Part model, mm, in its own coordinate system. Give positions to 0.01 mm unless a question says otherwise; leave off trailing zeros. Order: outer loops, then holes, each group sorted by start corner. A loop starts at its lowest first (then second) coordinate and runs counter-clockwise, first axis right, second up.
1. Slice it at A-A on z = 26. List the corners of the cut face in (x, y).
2. Drop flat-ended pins along their axis: pin 1 Ø6 at (y, z) = (5, 26) entering from +X; pin 2 Ø3.5 at (x, z) = (3, 231.5) entering from -Y. Give the stop position or say it passes through.
3. Slice it at B-B on z = 69. List the corners of the cut face in (x, y).
4. Probe line 1 (Y direction, x = 2.5, z = 133.5); line 2 (X direction, y = 5.25, z = 132); line 3 (Y direction, x = -1.3, z = 284). List the from-to ranges inside material, lowest first.
from build123d import *

# Parameters (mm, degrees)
BOSS_EXTRUDE1_DEPTH  = 310
SKETCH2_R            = 2.5
CUT_EXTRUDE1_DEPTH   = 311.25795719
CONVERT_SOLID2_DEPTH = 310


# Read off the part's stored shape, not the designer's step: Convert-Solid2
with BuildPart() as part:
    # Sketch1 → Boss-Extrude1 (new body)
    with BuildSketch(Plane.XY):
        Polygon((0, 0), (0, 10), (4, 10), (4, 12), (-2, 12), (-2, 0), align=None)
    extrude(amount=BOSS_EXTRUDE1_DEPTH)

    # Sketch2 → Cut-Extrude1 (cut, through all)
    with BuildSketch(Plane(origin=(0, 0, 0), x_dir=(0, 0, -1), z_dir=(1, 0, 0))):
        with Locations((-284, 5)):
            Circle(SKETCH2_R)
        with Locations((-198, 5)):
            Circle(SKETCH2_R)
        with Locations((-112, 5)):
            Circle(SKETCH2_R)
        with Locations((-26, 5)):
            Circle(SKETCH2_R)
    extrude(amount=-CUT_EXTRUDE1_DEPTH, mode=Mode.SUBTRACT)

    # Convert-Solid2 outline → Convert-Solid2 (cut)
    with BuildSketch(Plane.XY):
        with BuildLine():
            Line((-2, 12), (-2, 9))
            ThreePointArc((-2, 9), (-1.121320344, 11.121320344), (1, 12))
            Line((1, 12), (-2, 12))
        make_face()
        with BuildLine():
            Line((-1, 9), (-1, 0))
            Line((-1, 0), (0, 0))
            Line((0, 0), (0, 10))
            Line((0, 10), (4, 10))
            Line((4, 10), (4, 11))
            Line((4, 11), (1, 11))
            ThreePointArc((1, 11), (-0.414213562, 10.414213562), (-1, 9))
        make_face()
    extrude(amount=CONVERT_SOLID2_DEPTH, mode=Mode.SUBTRACT)


solid = part.part
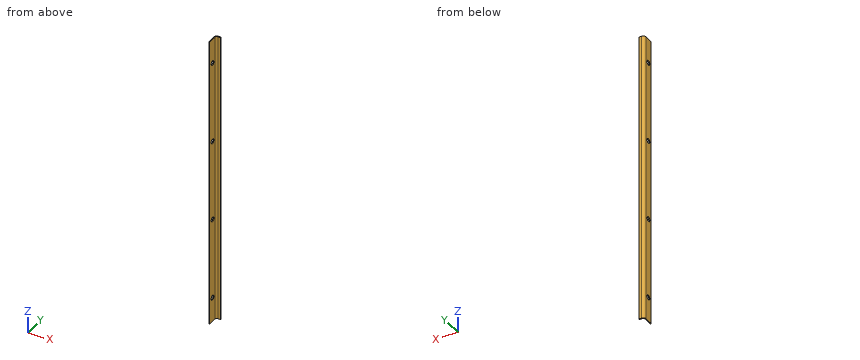
Data:
1. outline: (-2, 0) - (-1, 0) - (-1, 2.5) - (-2, 2.5) - close; (-2, 7.5) - (-1, 7.5) - (-1, 9) arc R2 cw to (1, 11) - (4, 11) - (4, 12) - (1, 12) arc R3 ccw to (-2, 9) - close
2. pin 1: stops at x = -1
2. pin 2: stops at y = 11
3. outline: (-2, 0) - (-1, 0) - (-1, 9) arc R2 cw to (1, 11) - (4, 11) - (4, 12) - (1, 12) arc R3 ccw to (-2, 9) - close
4. line 1: y = 11 to 12
4. line 2: x = -2 to -1
4. line 3: y = 0 to 2.5, 7.5 to 10.93
